Read the model definition and answer for the solid it produces. Units are mm, in the model's axes. Face numbers are marked on the shaded views. A direction names the side the tool comes from. Give positions to 0.01 mm unless a question says otherwise; leave off trailing zeros. Order: outer loops, then holes, each group sorted by start corner. A loop starts at its lowest first (then second) coordinate and runs counter-clockwise, first axis right, second up. Notation, with made-up numbers: (18, 11.25) - (24, 11.25) arc R7 cw to (24, 16.25) - close; hole circle Ø8 at (18, 81). An arc over 180 degrees is marked (long way). Write each question's results on one line, items separated by ' | '.
from build123d import *

# Parameters (mm, degrees)
SKETCH1_W           = 17.7
SKETCH1_H           = 43
BOSS_EXTRUDE1_DEPTH = 3
SKETCH2_W           = 3
SKETCH2_H           = 21.75
CUT_EXTRUDE1_DEPTH  = 56.240991234
CUT_EXTRUDE2_DEPTH  = 56.240991234
CUT_EXTRUDE3_DEPTH  = 2
SKETCH5_W           = 11.7
SKETCH5_H           = 16.5
BOSS_EXTRUDE2_DEPTH = 2
SKETCH6_W           = 9.3
SKETCH6_H           = 15.3
CUT_EXTRUDE4_DEPTH  = 2


with BuildPart() as part:
    # Sketch1 → Boss-Extrude1 (new body)
    with BuildSketch(Plane.XY):
        with Locations((-34.564285714, 12.525974026)):
            Rectangle(SKETCH1_W, SKETCH1_H)
    extrude(amount=BOSS_EXTRUDE1_DEPTH)

    # Sketch2 → Cut-Extrude1 (cut, through all)
    with BuildSketch(Plane.XY.offset(3)):
        with Locations((-41.914285714, 1.900974026)):
            Rectangle(SKETCH2_W, SKETCH2_H)
        with Locations((-27.214285714, 1.900974026)):
            Rectangle(SKETCH2_W, SKETCH2_H)
    extrude(amount=-CUT_EXTRUDE1_DEPTH, mode=Mode.SUBTRACT)

    # Sketch3 → Cut-Extrude2 (cut, through all)
    with BuildSketch(Plane.XY.offset(3)):
        with BuildLine():
            Line((-28.714285714, 25.525974026), (-38.714285714, 25.525974026))
            ThreePointArc((-38.714285714, 25.525974026), (-39.964285714, 26.775974026), (-38.714285714, 28.025974026))
            Line((-38.714285714, 28.025974026), (-28.714285714, 28.025974026))
            ThreePointArc((-28.714285714, 28.025974026), (-27.464285714, 26.775974026), (-28.714285714, 25.525974026))
        make_face()
    extrude(amount=-CUT_EXTRUDE2_DEPTH, mode=Mode.SUBTRACT)

    # Sketch4 → Cut-Extrude3 (cut)
    with BuildSketch(Plane.XY.offset(3)):
        with BuildLine():
            Line((-38.714285714, 28.775974026), (-28.714285714, 28.775974026))
            ThreePointArc((-28.714285714, 28.775974026), (-26.714285714, 26.775974026), (-28.714285714, 24.775974026))
            Line((-28.714285714, 24.775974026), (-38.714285714, 24.775974026))
            ThreePointArc((-38.714285714, 24.775974026), (-40.714285714, 26.775974026), (-38.714285714, 28.775974026))
        make_face()
    extrude(amount=-CUT_EXTRUDE3_DEPTH, mode=Mode.SUBTRACT)

    # Sketch5 → Boss-Extrude2 (add)
    with BuildSketch(Plane.XY.offset(3)):
        with Locations((-34.564285714, -0.724025974)):
            Rectangle(SKETCH5_W, SKETCH5_H)
    extrude(amount=BOSS_EXTRUDE2_DEPTH)

    # Sketch6 → Cut-Extrude4 (cut)
    with BuildSketch(Plane.XY.offset(5)):
        with Locations((-34.564285714, -1.324025974)):
            Rectangle(SKETCH6_W, SKETCH6_H)
    extrude(amount=-CUT_EXTRUDE4_DEPTH, mode=Mode.SUBTRACT)


solid = part.part
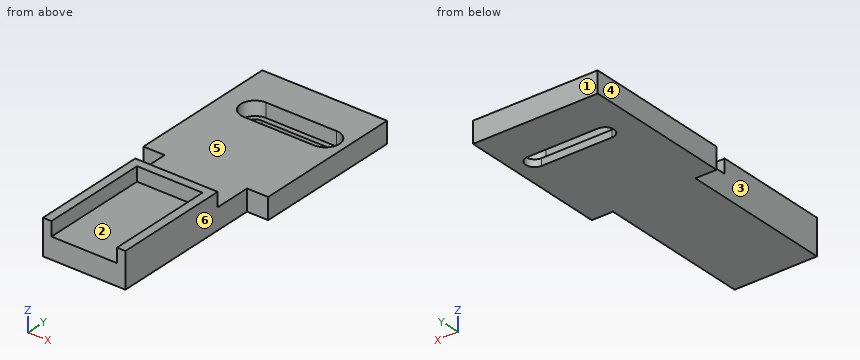
(1) Section A-A (x = -36.5) is taken. Give the vertices of the cut face in (y, z), plus the area to 3 significant figures.
Conclusion:
outline: (-8.97, 0) - (25.53, 0) - (25.53, 1) - (24.78, 1) - (24.78, 3) - (7.53, 3) - (7.53, 5) - (6.33, 5) - (6.33, 3) - (-8.97, 3) - close; (28.03, 0) - (34.03, 0) - (34.03, 3) - (28.78, 3) - (28.78, 1) - (28.03, 1) - close | area: 121 mm^2
(2) Section B-B (z = 2) is taken. Give the vertices of the cut face in (x, y), plus the area to 3 significant figures.
Conclusion:
outline: (-43.41, 12.78) - (-40.41, 12.78) - (-40.41, -8.97) - (-28.71, -8.97) - (-28.71, 12.78) - (-25.71, 12.78) - (-25.71, 34.03) - (-43.41, 34.03) - close; hole (-38.71, 24.78) - (-28.71, 24.78) arc R2 ccw to (-28.71, 28.78) - (-38.71, 28.78) arc R2 ccw to start | area: 578 mm^2
(3) Section C-C (y = -1) is taken. Give the vertices of the cut face in (x, z).
Conclusion:
outline: (-40.41, 0) - (-28.71, 0) - (-28.71, 5) - (-29.91, 5) - (-29.91, 3) - (-39.21, 3) - (-39.21, 5) - (-40.41, 5) - close
(4) Consider probe 1 along Y at (x, z) = (-35.25, 0.3); probe 2 along X at (y, z) = (-4.5, 3.9); probe 3 along Y at (x, z) = (-30, 1.7). Determine where each line is inside the solid, lowest interval first. Write a range as [from, to].
Conclusion:
probe 1: [-8.97, 25.53], [28.03, 34.03] | probe 2: [-40.41, -39.21], [-29.91, -28.71] | probe 3: [-8.97, 24.78], [28.78, 34.03]
(5) Each of these flat-tipped pins is pushed along its axis until it touches: pin 1 (2.5 mm diameter, centred on y = 7, z = 1.5, fed in from +X); pin 2 (1.6 mm diameter, centred on x = -35, z = 4.5, fed in from +Y); pin 3 (1 mm diameter, centred on y = 1.5, z = 4, fed in from -X). Where does it stop, or does it pass through?
Conclusion:
pin 1: x = -28.71 | pin 2: y = 7.53 | pin 3: x = -40.41
(6) The mould has two halves that part along X. Classify the marked faces 1, 2 and 3: pulls with the +X half, pulls with the -X half, needs draft (parallel to the pull), parting line crosses it, or undercut.
Conclusion:
face 1: needs draft | face 2: undercut | face 3: pulls with the -X half
(7) For the marked faces 4, 5 and 6, determine the directions among +Z, -Z, +X, -X, +Y, -Y from which every point of the face is accessible in a straight line to the end or side of a thin tool.
Conclusion:
face 4: +Z, -Z, -X, +Y, -Y | face 5: +Z, +X, -X, +Y | face 6: +Z, -Z, +X, -Y
(8) Section D-D (z = 4.1) is taken. Give the vertices of the cut face in (x, y), plus the area to 3 significant figures.
Conclusion:
outline: (-40.41, -8.97) - (-39.21, -8.97) - (-39.21, 6.33) - (-29.91, 6.33) - (-29.91, -8.97) - (-28.71, -8.97) - (-28.71, 7.53) - (-40.41, 7.53) - close | area: 50.8 mm^2
